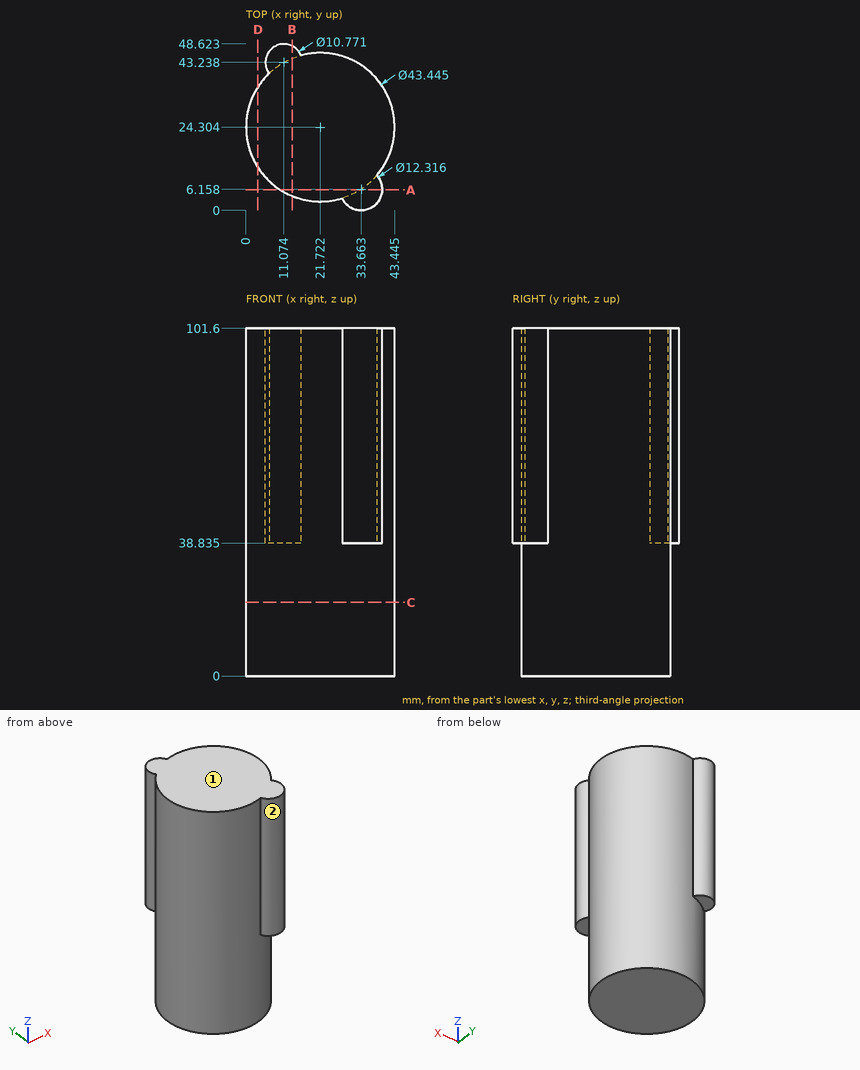
Source: three-view drawing plus pictorial views. Frame: mm from the lowest corner of the part. Round coordinates to 2 decimals unless told otherwise and drop trailing zeros. Write each loop counter-clockwise with the first axis right and the second up, starting at its lowest first coordinate (ties: lowest second). Pieces come first, ordered by that corner, then holes. Notation, with made-up numbers: (89, -12) -> (132, -12) arc R35 cw to (132, 25) -> close; hole circle Ø6 at (29, 15). An arc over 180 degrees is marked (long way). Return JSON: item names as keys, results as strings.
Q1. Section B-B on x = 13.5. Return the cut outline in (y, z) (1 decimal).
From the geometry:
{"outline": "(4.2, 0) -> (44.4, 0) -> (44.4, 38.8) -> (48, 38.8) -> (48, 101.6) -> (4.2, 101.6) -> close"}
Q2. Section D-D on x = 3.5. Return the cut outline in (y, z), and give its area (3 significant figures).
From the geometry:
{"outline": "(12.48, 0) -> (36.13, 0) -> (36.13, 101.6) -> (12.48, 101.6) -> close", "area": "2,400 mm2"}
Q3. First-contact query: pin 1 Ø1 at (y, z) = (6, 80.5) entering from -X; pin 2 Ø1.5 at (x, z) = (7.5, 18.5) entering from +Y (1 decimal); pin 3 Ø1.5 at (y, z) = (39, 55.5) entering from +X; pin 4 Ø6 at (x, y) = (30.5, 18.5) entering from -Z. Flat tips, straight axial feed; report the tip coordinate or a pass-through.
From the geometry:
{"pin 1": "x = 9.28", "pin 2": "y = 41.3", "pin 3": "x = 38.38", "pin 4": "z = 0"}
Q4. Ray query, line 1 (Y direction, x = 21, z = 75) (1 decimal); line 2 (X direction, y = 25, z = 5.5); line 3 (Y direction, x = 33, z = 71.5) (1 decimal). Return the intervals inside material, ascending.
From the geometry:
{"line 1": "2.6 to 46", "line 2": "0.01 to 43.43", "line 3": "0 to 42.9"}
Q5. Section C-C on z = 21.5. Return the cut outline in (x, y) (1 decimal), and give its area (3 significant figures).
From the geometry:
{"outline": "circle Ø43.4 at (21.7, 24.3)", "area": "1,480 mm2"}
Q6. Section A-A on y = 6. Return the cut outline in (x, z) (1 decimal).
From the geometry:
{"outline": "(10, 0) -> (33.4, 0) -> (33.4, 38.8) -> (39.8, 38.8) -> (39.8, 101.6) -> (10, 101.6) -> close"}
Q7. Mould query, pull axis Y, two halves, no side actions, for the marked faces 1 and 2. Classes: +Y half, -Y half, draft (parallel to the pull), parting line (faces both ways), or undercut.
From the geometry:
{"face 1": "draft", "face 2": "undercut"}
